Autodesk Inventor part; units mm, degrees
ref_plane "Work Plane1" through (0, 0, -4) normal (0, 0, 1) x (1, 0, 0)
ref_plane "YZ Plane" through (0, 0, 0) normal (1, 0, 0) x (0, 1, 0)
ref_plane "XZ Plane" through (0, 0, 0) normal (0, 1, 0) x (-1, 0, 0)
sketch "Sketch1" plane through (0, 0, 0) normal (0, 0, 1) x (1, 0, 0)
  line L0 (7, 0) -> (47, 0)
  line L1 (47, 20) -> (7, 20)
  line L2 (7, 20) -> (7, 0)
  line L3 (47, 20) -> (47, 0)
  point P0 (0, 0)
extrude "Extrusion1" add sketch "Sketch1" along normal blind 28 and the other way blind 10
sketch "Sketch2" plane through (0, 0, -10) normal (0, 0, -1) x (-1, 0, 0)
  line L0 (-7, 20) -> (-47, 20)
  line L1 (-47, 20) -> (-47, 10)
  line L2 (-47, 20) -> (-47, 0)
  line L3 (-47, 10) -> (-37, 10)
  circle A0 centre (-37, 10) radius 2.5
  point P0 (0, 0)
  dimension "d10" = 10
  dimension "d11" = 10
  dimension "d12" = 5
extrude "Extrusion3" add sketch "Sketch2" along normal blind 8
sketch "Sketch3" plane through (0, 0, -10) normal (0, 0, -1) x (-1, 0, 0)
  circle A0 centre (-37, 10) radius 2.5
  circle A1 centre (-37, 10) radius 10
  line L0 (-47, 20) -> (-7, 20)
  line L1 (-7, 20) -> (0, 20)
  line L2 (-7, 20) -> (-12, 20)
  line L3 (-7, 20) -> (-47, 20)
  line L4 (-12, 20) -> (-12, 0)
  line L5 (-7, 0) -> (-47, 0)
  line L6 (-47, 0) -> (-7, 0)
  point P0 (0, 0)
  point P1 (-37, 0)
  point P2 (-37, 20)
  dimension "d15" = 5
extrude "Extrusion4" add sketch "Sketch3" along normal blind 1
ref_plane "Work Plane1" through (0, 0, -4) normal (0, 0, 1) x (1, 0, 0)
sketch "Sketch4" plane through (0, 0, -4) normal (0, 0, 1) x (1, 0, 0)
  line L0 (47, 0) -> (47, 20)
  line L1 (47, 20) -> (54, 20)
  line L2 (54, 0) -> (47, 0)
  line L3 (47, 20) -> (7, 20)
  line L4 (47, 0) -> (47, 20)
  line L5 (7, 20) -> (7, 0)
  line L6 (7, 0) -> (0, 0)
  line L7 (0, 20) -> (7, 20)
  line L8 (7, 10) -> (7, 15)
  line L9 (7, 15) -> (2, 15)
  arc A0 (0, 13.5) -> (0, 16.5) centre (2, 15) ccw
  line L10 (27, 10) -> (22.2315, 10)
  line L11 (47, 20) -> (47, 10)
  line L12 (47, 20) -> (27, 20)
  line L13 (27, 20) -> (27, 13.3752)
  arc A1 (0, 3.5) -> (0, 6.5) centre (2, 5) ccw
  arc A2 (54, 16.5) -> (54, 13.5) centre (52, 15) ccw
  arc A3 (54, 6.5) -> (54, 3.5) centre (52, 5) ccw
  line L14 (54, 20) -> (54, 16.5)
  line L15 (54, 13.5) -> (54, 6.5)
  line L16 (54, 3.5) -> (54, 0)
  line L17 (0, 0) -> (0, 3.5)
  line L18 (0, 6.5) -> (0, 13.5)
  line L19 (0, 16.5) -> (0, 20)
  dimension "d19" = 7
  dimension "d21" = 7
  dimension "d22" = 5
  dimension "d23" = 5
  dimension "d24" = 5
  dimension "d25" = 20
extrude "Extrusion5" add sketch "Sketch4" along normal blind 2.5
sketch "Sketch5" plane through (0, 0, -11) normal (0, 0, -1) x (-1, 0, 0)
  circle A0 centre (-37, 10) radius 2.5
  circle A1 centre (-37, 10) radius 2.5
  circle A2 centre (-37, 10) radius 6.5
  point P0 (0, 0)
  dimension "d28" = 13
extrude "Extrusion6" add sketch "Sketch5" along normal blind 2
sketch "Sketch6" plane through (47, 0, 28) normal (1, 0, 0) x (0, 0, -1)
  line L0 (29.5, 0) -> (0, 0)
  line L1 (0, 0) -> (10, 0)
  line L2 (10, 0) -> (10, 20)
  line L3 (0, 20) -> (29.5, 20)
  line L4 (0, 20) -> (10, 20)
  line L5 (0, 0) -> (0, 20)
  point P0 (28, 0)
  dimension "d31" = 10
extrude "Extrusion7" add sketch "Sketch6" along normal blind 10
properties part number "Motorv2"
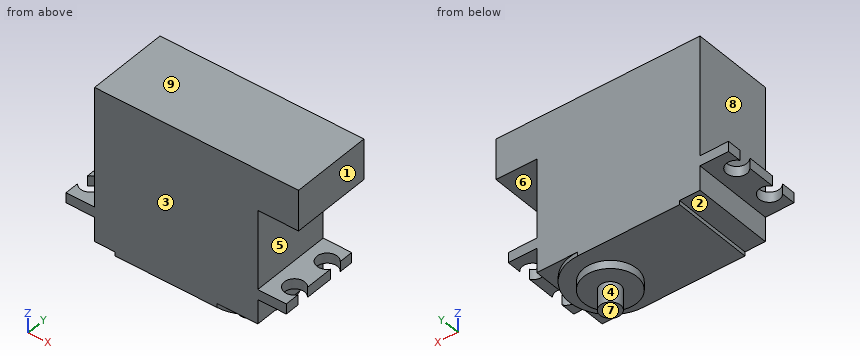
The listing builds one solid part. Answer for the finished solid, in the listing's coordinates (mm). Face numbers are marked on the shaded views. A direction names the side the tool comes from. Round coordinates to 2 decimals unless told otherwise and drop trailing zeros. Order: outer loops, then holes, each group sorted by start corner. A loop starts at its lowest first (then second) coordinate and runs counter-clockwise, first axis right, second up. Notation, with made-up numbers: (15, 16) -> (31, 16) arc R31 ccw to (31, 53) -> close; hole circle Ø10 at (61.25, 14). An arc over 180 degrees is marked (long way). Put each result on its own line as item: value.
Q1. Determine the mould class of the marked faces 6, 7, 8 and 9 for opening direction Z: pulls with the +Z half, pulls with the -Z half, needs draft (parallel to the pull), parting line crosses it, or undercut.
Results list:
face 6: undercut
face 7: pulls with the -Z half
face 8: needs draft
face 9: pulls with the +Z half
Q2. Consider line 1 along Y through (x, z) = (52, -3.3); line 2 along Z through (x, y) = (53, 12.5); line 3 along Z through (x, y) = (34.5, 1.25). Determine where each line is inside the solid, lowest interval first.
Results list:
line 1: 0 to 2.5, 7.5 to 12.5, 17.5 to 20
line 2: -4 to -1.5, 18 to 28
line 3: -11 to 28
Q3. Section A-A, the plane x = 2 is taken. Write down the section's boundary in (y, z).
Results list:
outline: (0, -4) -> (2.5, -4) -> (2.5, -1.5) -> (0, -1.5) -> close; (7.5, -4) -> (12.5, -4) -> (12.5, -1.5) -> (7.5, -1.5) -> close; (17.5, -4) -> (20, -4) -> (20, -1.5) -> (17.5, -1.5) -> close
Q4. Section C-C, the plane y = 1 is taken. Write down the section's boundary in (x, z).
Results list:
outline: (0, -4) -> (7, -4) -> (7, -10) -> (12, -10) -> (12, -11) -> (41.36, -11) -> (41.36, -10) -> (47, -10) -> (47, -4) -> (54, -4) -> (54, -1.5) -> (47, -1.5) -> (47, 18) -> (57, 18) -> (57, 28) -> (7, 28) -> (7, -1.5) -> (0, -1.5) -> close
Q5. Each of these flat-tipped pins is pushed along its axis until it touches: P1, Ø5.5, axis at x = 10, y = 12.5, coming from the -Z side; P2, Ø4, axis at x = 2, y = 15, coming from the -Z side; P3, Ø5, axis at y = 14, z = 15, coming from the +X side; P4, Ø5, axis at x = 42, y = 4.5, coming from the -Z side. Where does it stop, or does it pass through?
Results list:
P1: z = -11
P2: through
P3: x = 47
P4: z = -13
Q6. Section D-D, the plane x = 25 is taken. Write down the section's boundary in (y, z).
Results list:
outline: (0, -11) -> (20, -11) -> (20, 28) -> (0, 28) -> close
Q7. Which of the six approach directions +Z, -Z, +X, -X, +Y, -Y give full straight-line access (tool end or side, diameter ignored) to the marked faces 1, 2, 3, 4 and 5?
Results list:
face 1: +Z, -Z, +X, +Y, -Y
face 2: -Z, -X, +Y, -Y
face 3: +Z, -Z, +X, -X, -Y
face 4: -Z
face 5: +X, +Y, -Y
Q8. Section B-B, the plane z = 2.5 is taken. Write down the section's boundary in (x, y).
Results list:
outline: (7, 0) -> (47, 0) -> (47, 20) -> (7, 20) -> close
